```python
from build123d import *

# Parameters (mm, degrees)
F1_DEPTH = 30
F2_SIZE  = 5
F3_R     = 15
F4_R     = 17.5
F5_DEPTH = 40
F6_SIZE  = 5


with BuildPart() as f1:
    # F0 (on Top) → F1 (new body)
    with BuildSketch(Plane.XY):
        Polygon((22.451399, 30.901699), (0, 100), (-22.451399, 30.901699), (-95.105652, 30.901699), (-36.327126, -11.803399), (-58.778525, -80.901699), (0, -38.196601), (58.778525, -80.901699), (36.327126, -11.803399), (95.105652, 30.901699), align=None)
    extrude(amount=F1_DEPTH)

    # F2
    f2_edges = [f1.edges().sort_by_distance(p)[0] for p in [
        (65.716389, 9.54915, 30),
        (58.778525, 30.901699, 30),
        (11.225699, 65.45085, 30),
        (-11.225699, 65.45085, 30),
        (-58.778525, 30.901699, 30),
        (-65.716389, 9.54915, 30),
        (-47.552826, -46.352549, 30),
        (-29.389263, -59.54915, 30),
        (29.389263, -59.54915, 30),
        (47.552826, -46.352549, 30),
    ]]
    chamfer(f2_edges, length=F2_SIZE)

    # F3
    f3_edges = [f1.edges().sort_by_distance(p)[0] for p in [
        (65.716389, 9.54915, 0),
        (58.778525, 30.901699, 0),
        (11.225699, 65.45085, 0),
        (-11.225699, 65.45085, 0),
        (-58.778525, 30.901699, 0),
        (-65.716389, 9.54915, 0),
        (-47.552826, -46.352549, 0),
        (-29.389263, -59.54915, 0),
        (29.389263, -59.54915, 0),
        (47.552826, -46.352549, 0),
    ]]
    fillet(f3_edges, radius=F3_R)

    # F4 (on face) → F5 (cut)
    with BuildSketch(Plane(origin=(0, 0, 0), x_dir=(1, 0, 0), z_dir=(0, 0, -1))):
        Circle(F4_R)
    extrude(amount=-F5_DEPTH, mode=Mode.SUBTRACT)

    # F6
    f6_edges = [f1.edges().sort_by_distance(p)[0] for p in [
        (-17.5, 0, 30),
    ]]
    chamfer(f6_edges, length=F6_SIZE)


solid = f1.part
```
Here's how the part is built. I have some questions about the finished solid (model axes, mm). A direction names the side the tool comes from. Coordinates: 2 decimals unless noted, no trailing zeros. Write each loop counter-clockwise with the first axis right and the second up, starting at its lowest first coordinate (ties: lowest second). Pieces come first, ordered by that corner, then holes. Notation, with made-up numbers: (25.25, 25) -> (42.25, 25) arc R13 cw to (42.25, 46) -> close; hole circle Ø5 at (-35.75, -29). An arc over 180 degrees is marked (long way). Use a Markdown table: item, result. Add a question column.
(1) Please list where these lines run through material, in increasing order: line 1 (X direction, y = -39.5, z = 24); line 2 (X direction, y = 11.5, z = 13); line 3 (X direction, y = 42, z = 19.5).
(2) We'd pull the mould along X, two halves only. Please class faces 1 (the flat face through (-58, 30.902, 20)), 2 (the cylindrical face through (43.018, -41.482, 6.262)), 3 (the flat face through (28.98, -59.25, 19.93)), 4 (the cylindrical face through (-13.887, 10.648, 12.325)): +X half, -X half, draft (parallel to the pull), parting line (faces both ways), or undercut.
(3) For faces 5 (the cylindrical face through (60.13, 8.96, 6.26)), 6 (the flat face through (57.5, 28.4, 27.5)), 7 (the flat face through (47.7, -46.8, 19.9)), 8 (the flat face through (-66.13, 9.85, 19.93)), which set-ups out of +Z, -Z, +X, -X, +Y, -Y let a thin tool reach every point of the face, with its end or its side?
(4) I'm going to push flat-ended pins straight in: P1, Ø10, axis at x = 1, z = 13, coming from the -Y side; P2, Ø4, axis at y = 17, z = 19.5, coming from the -X side; P3, Ø5, axis at x = 56.5, z = 22, coming from the +Y side. Where does each tip first touch, or does it pass through?
(5) If we section it at A-A, the plane z = 9.5: Write out the boundary of the cut face in (x, y), and give its area (3 significant figures).
Outcome:
| question | item | result |
|---|---|---|
| 1 | line 1 | x = -45.33 to -1.79, 1.79 to 45.33 |
| 1 | line 2 | x = -68.17 to -13.19, 13.19 to 68.17 |
| 1 | line 3 | x = -18.85 to 18.85 |
| 2 | face 1 | draft |
| 2 | face 2 | +X half |
| 2 | face 3 | undercut |
| 2 | face 4 | undercut |
| 3 | face 5 | -Z, +X |
| 3 | face 6 | +Z, +X, +Y |
| 3 | face 7 | +Z, -Z, +X |
| 3 | face 8 | +Z, -Z, -X |
| 4 | P1 | stops at y = -42.45 |
| 4 | P2 | stops at x = -78.72 |
| 4 | P3 | stops at y = 30.9 |
| 5 | outline | (-91.89, 29.86) -> (-35.1, -11.4) -> (-56.79, -78.17) -> (0, -36.91) -> (56.79, -78.17) -> (35.1, -11.4) -> (91.89, 29.86) -> (21.69, 29.86) -> (0, 96.62) -> (-21.69, 29.86) -> close; hole circle Ø35 at (0, 0) |
| 5 | area | 9,520 mm^2 |
